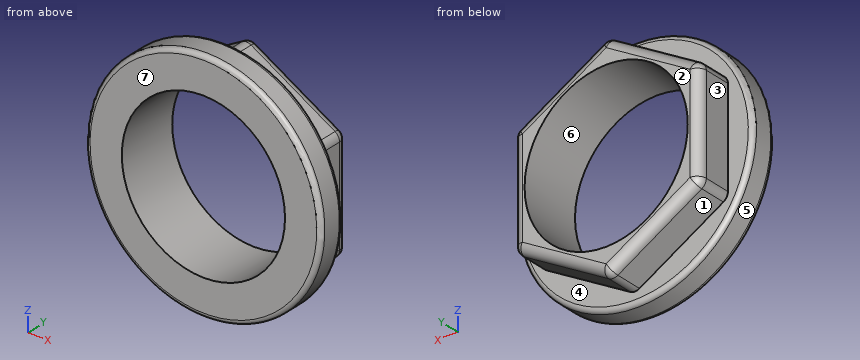
from build123d import *

# Parameters (mm, degrees)
ESQUISSE1_R        = 13
ESQUISSE1_R_2      = 9
BOSS_EXTRU_1_DEPTH = 3
ESQUISSE2_R        = 9
BOSS_EXTRU_2_DEPTH = 4
CONG_2_R           = 1
CONG_3_R           = 0.5


with BuildPart() as part:
    # Esquisse1 → Boss.-Extru.1 (new body)
    with BuildSketch(Plane(origin=(0, 0, 0), x_dir=(1, 0, 0), z_dir=(0, 1, 0))):
        with Locations(Location((0, 0, 0), (0, 0, 270))):
            Circle(ESQUISSE1_R)
        with Locations(Location((0, 0, 0), (0, 0, 270))):
            Circle(ESQUISSE1_R_2, mode=Mode.SUBTRACT)
    extrude(amount=BOSS_EXTRU_1_DEPTH)

    # Esquisse2 → Boss.-Extru.2 (add)
    with BuildSketch(Plane(origin=(0, 3, 0), x_dir=(1, 0, 0), z_dir=(0, 1, 0))):
        Polygon((10.25, -5.917840259), (10.25, 5.917840259), (0, 11.835680518), (-10.25, 5.917840259), (-10.25, -5.917840259), (0, -11.835680518), align=None)
        with Locations(Location((0, 0, 0), (0, 0, 270))):
            Circle(ESQUISSE2_R, mode=Mode.SUBTRACT)
    extrude(amount=BOSS_EXTRU_2_DEPTH)

    # Congé2
    cong_2_edges = [part.edges().sort_by_distance(p)[0] for p in [
        (5.125, 7, 8.876760389),
        (10.25, 7, 0),
        (5.125, 7, -8.876760389),
        (-5.125, 7, -8.876760389),
        (-10.25, 7, 0),
        (-5.125, 7, 8.876760389),
        (0, 5, 11.835680518),
        (10.25, 5, 5.917840259),
        (10.25, 5, -5.917840259),
        (0, 5, -11.835680518),
        (-10.25, 5, -5.917840259),
        (-10.25, 5, 5.917840259),
    ]]
    fillet(cong_2_edges, radius=CONG_2_R)

    # Congé3
    cong_3_edges = [part.edges().sort_by_distance(p)[0] for p in [
        (0, 0, -13),
        (0, 3, -13),
    ]]
    fillet(cong_3_edges, radius=CONG_3_R)


solid = part.part
Input: part model. Units: mm. Frame: model coordinates. Face numbers are marked on the shaded views. A direction names the side the tool comes from. Round coordinates to 2 decimals unless told otherwise and drop trailing zeros. Loops run counter-clockwise (first coordinate to the right, second up) from the corner with the lowest first, then second, coordinate; pieces in that order, holes last. Notation, with made-up numbers: (61.25, 15) -> (115.25, 15) arc R26 ccw to (115.25, 40) -> close; hole circle Ø8 at (-12.75, -17.5). An arc over 180 degrees is marked (long way). Answer as a JSON object with one key per item and string values. Group by question number.
1) Section query A-A on y = 4.75. Output: boundary loops of the cut face in (x, z), plus the area to 3 significant figures.
2) Reachability of the marked faces 1, 2, 3 and 4 from +Z, -Z, +X, -X, +Y, -Y: full face, straight path, thin tool, end or side. Return the list, or none.
3) Section query C-C on y = 6.5. Output: boundary loops of the cut face in (x, z), plus the area to 3 significant figures.
4) Ray query, L1, parallel to X at y = 4.5, z = 0; L2, parallel to X at y = 1.5, z = 0; L3, parallel to Y at x = -6, z = 10. Return the intervals inside material, ascending.
5) Section query B-B on z = 0. Output: boundary loops of the cut face in (x, y), plus the area to 3 significant figures.
6) Pin query (flat end, axial travel): pin 1 (4 mm diameter, centred on x = 7.5, y = 5.5, fed in from -Z); pin 2 (2 mm diameter, centred on x = 7, y = 5, fed in from +Z); pin 3 (1 mm diameter, centred on x = -1.5, y = 5, fed in from -Z). Return the tip coordinate at first contact, or that it passes through.
7) Draft query along Z for the marked faces 5, 6 and 7. Return one class per face: +Z half, -Z half, draft (parallel to the pull), parting line (faces both ways), or undercut.
8) Section query D-D on y = 1. Output: boundary loops of the cut face in (x, z).
Reply:
{
 "1": {"outline": "(-10.25, -5.34) arc R1 ccw to (-9.75, -6.21) -> (-0.5, -11.55) arc R1 ccw to (0.5, -11.55) -> (9.75, -6.21) arc R1 ccw to (10.25, -5.34) -> (10.25, 5.34) arc R1 ccw to (9.75, 6.21) -> (0.5, 11.55) arc R1 ccw to (-0.5, 11.55) -> (-9.75, 6.21) arc R1 ccw to (-10.25, 5.34) -> close; hole circle Ø18 at (0, 0)", "area": "109 mm2"},
 "2": {"face 1": "-Z, -X, +Y", "face 2": "+Z, -Z, +X, -X, +Y", "face 3": "+Z, -Z, -X, +Y", "face 4": "+Y"},
 "3": {"outline": "(-10.12, -5.34) arc R0.87 ccw to (-9.68, -6.09) -> (-0.43, -11.43) arc R0.87 ccw to (0.43, -11.43) -> (9.68, -6.09) arc R0.87 ccw to (10.12, -5.34) -> (10.12, 5.34) arc R0.87 ccw to (9.68, 6.09) -> (0.43, 11.43) arc R0.87 ccw to (-0.43, 11.43) -> (-9.68, 6.09) arc R0.87 ccw to (-10.12, 5.34) -> close; hole circle Ø18 at (0, 0)", "area": "99.8 mm2"},
 "4": {"L1": "x = -10.25 to -9, 9 to 10.25", "L2": "x = -13 to -9, 9 to 13", "L3": "y = 0 to 3"},
 "5": {"outline": "(-13, 0.5) arc R0.5 ccw to (-12.5, 0) -> (-9, 0) -> (-9, 7) -> (-9.25, 7) arc R1 ccw to (-10.25, 6) -> (-10.25, 3) -> (-12.5, 3) arc R0.5 ccw to (-13, 2.5) -> close; (9, 0) -> (12.5, 0) arc R0.5 ccw to (13, 0.5) -> (13, 2.5) arc R0.5 ccw to (12.5, 3) -> (10.25, 3) -> (10.25, 6) arc R1 ccw to (9.25, 7) -> (9, 7) -> close", "area": "33.4 mm2"},
 "6": {"pin 1": "stops at z = -8.66", "pin 2": "stops at z = 8.37", "pin 3": "stops at z = -11.26"},
 "7": {"face 5": "parting line", "face 6": "undercut", "face 7": "draft"},
 "8": {"outline": "circle Ø26 at (0, 0); hole circle Ø18 at (0, 0)"}
}
